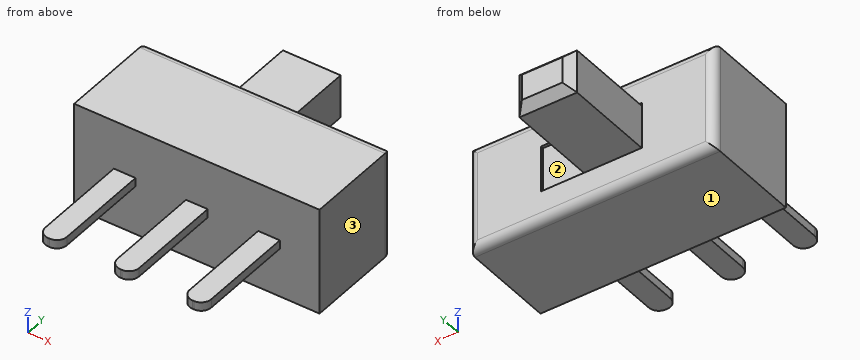
```python
from build123d import *

# Parameters (mm, degrees)
SKETCH1_W           = 8.5
SKETCH1_H           = 3.7
BOSS_EXTRUDE1_DEPTH = 1.75
SKETCH2_W           = 3.5
SKETCH2_H           = 1.6
CUT_EXTRUDE1_DEPTH  = 0.1
SKETCH3_W           = 2
SKETCH3_H           = 1.5
BOSS_EXTRUDE2_DEPTH = 3.5
SKETCH4_W           = 0.75
SKETCH4_H           = 0.3
BOSS_EXTRUDE3_DEPTH = 3.7
CHAMFER1_SIZE       = 0.3
FILLET1_R           = 0.3
FILLET2_R           = 0.35


with BuildPart() as part:
    # Sketch1 → Boss-Extrude1 (new, symmetric)
    with BuildSketch(Plane(origin=(0, 0, 0), x_dir=(1, 0, 0), z_dir=(0, 1, 0))):
        Rectangle(SKETCH1_W, SKETCH1_H)
    extrude(amount=BOSS_EXTRUDE1_DEPTH, both=True)

    # Sketch2 → Cut-Extrude1 (cut)
    with BuildSketch(Plane(origin=(0, 1.75, 0), x_dir=(1, 0, 0), z_dir=(0, 1, 0))):
        Rectangle(SKETCH2_W, SKETCH2_H)
    extrude(amount=-CUT_EXTRUDE1_DEPTH, mode=Mode.SUBTRACT)

    # Sketch3 → Boss-Extrude2 (add)
    with BuildSketch(Plane(origin=(0, 1.65, 0), x_dir=(1, 0, 0), z_dir=(0, 1, 0))):
        with Locations((-0.7, 0)):
            Rectangle(SKETCH3_W, SKETCH3_H)
    extrude(amount=BOSS_EXTRUDE2_DEPTH)

    # Sketch4 → Boss-Extrude3 (add)
    with BuildSketch(Plane.XZ.offset(1.75)):
        Rectangle(SKETCH4_W, SKETCH4_H)
        with Locations((-2.5, 0)):
            Rectangle(SKETCH4_W, SKETCH4_H)
        with Locations((2.5, 0)):
            Rectangle(SKETCH4_W, SKETCH4_H)
    extrude(amount=BOSS_EXTRUDE3_DEPTH)

    # Chamfer1
    chamfer1_edges = [part.edges().sort_by_distance(p)[0] for p in [
        (-1.7, 5.15, 0),
        (-0.7, 5.15, 0.75),
        (0.3, 5.15, 0),
        (-0.7, 5.15, -0.75),
    ]]
    chamfer(chamfer1_edges, length=CHAMFER1_SIZE)

    # Fillet1
    fillet1_edges = [part.edges().sort_by_distance(p)[0] for p in [
        (-4.25, 1.75, 0),
        (0, 1.75, 1.85),
        (4.25, 1.75, 0),
        (0, 1.75, -1.85),
    ]]
    fillet(fillet1_edges, radius=FILLET1_R)

    # Fillet2
    fillet2_edges = [part.edges().sort_by_distance(p)[0] for p in [
        (0.375, -5.45, 0),
        (-0.375, -5.45, 0),
        (-2.125, -5.45, 0),
        (-2.875, -5.45, 0),
        (2.125, -5.45, 0),
        (2.875, -5.45, 0),
    ]]
    fillet(fillet2_edges, radius=FILLET2_R)


solid = part.part
```
Design review of the part built by this model. Coordinates are the model's own, in mm. Face numbers are marked on the shaded views. Give positions to 0.01 mm unless a question says otherwise; leave off trailing zeros. Write each loop counter-clockwise with the first axis right and the second up, starting at its lowest first coordinate (ties: lowest second). Pieces come first, ordered by that corner, then holes. Notation, with made-up numbers: (74.5, 1) -> (94.5, 1) arc R22 ccw to (94.5, 35) -> close; hole circle Ø3 at (44, 44). An arc over 180 degrees is marked (long way). Answer in a Markdown table with one row per item.
(1) Consider section C-C (z = 0.6). State the section outline as (x, y) points.
Results:
| item | result |
|---|---|
| outline | (-4.25, -1.75) -> (4.25, -1.75) -> (4.25, 1.45) arc R0.3 ccw to (3.95, 1.75) -> (1.75, 1.75) -> (1.75, 1.65) -> (0.3, 1.65) -> (0.3, 4.85) -> (0.15, 5) -> (-1.55, 5) -> (-1.7, 4.85) -> (-1.7, 1.65) -> (-1.75, 1.65) -> (-1.75, 1.75) -> (-3.95, 1.75) arc R0.3 ccw to (-4.25, 1.45) -> close |
(2) Clearance check with flat-ended pins moving along their axes: pin 1 (0.6 mm diameter, centred on x = -1, y = 3, fed in from +Z); pin 2 (1.8 mm diameter, centred on x = -1, z = -0.5, fed in from -Y); pin 3 (0.6 mm diameter, centred on x = 2.5, y = -3, fed in from -Z). State where each tip first meets the part, or that it passes through.
Results:
| item | result |
|---|---|
| pin 1 | z = 0.75 |
| pin 2 | y = -5.42 |
| pin 3 | z = -0.15 |
(3) Consider section D-D (x = 0.75). State the section outline as (y, z) points.
Results:
| item | result |
|---|---|
| outline | (-1.75, -1.85) -> (1.45, -1.85) arc R0.3 ccw to (1.75, -1.55) -> (1.75, -0.8) -> (1.65, -0.8) -> (1.65, 0.8) -> (1.75, 0.8) -> (1.75, 1.55) arc R0.3 ccw to (1.45, 1.85) -> (-1.75, 1.85) -> close |
(4) Consider section B-B (x = -1.25). State the section outline as (y, z) points.
Results:
| item | result |
|---|---|
| outline | (-1.75, -1.85) -> (1.45, -1.85) arc R0.3 ccw to (1.75, -1.55) -> (1.75, -0.8) -> (1.65, -0.8) -> (1.65, -0.75) -> (4.85, -0.75) -> (5.15, -0.45) -> (5.15, 0.45) -> (4.85, 0.75) -> (1.65, 0.75) -> (1.65, 0.8) -> (1.75, 0.8) -> (1.75, 1.55) arc R0.3 ccw to (1.45, 1.85) -> (-1.75, 1.85) -> close |
(5) Consider section A-A (y = -2). State the section outline as (x, z) points (3 decimals).
Results:
| item | result |
|---|---|
| outline | (-2.875, -0.15) -> (-2.125, -0.15) -> (-2.125, 0.15) -> (-2.875, 0.15) -> close; (-0.375, -0.15) -> (0.375, -0.15) -> (0.375, 0.15) -> (-0.375, 0.15) -> close; (2.125, -0.15) -> (2.875, -0.15) -> (2.875, 0.15) -> (2.125, 0.15) -> close |
(6) Mouldability with a two-part tool opening along X and no side actions: class the marked faces 1, 2 and 3 as +X half, -X half, draft (parallel to the pull), parting line (faces both ways), or undercut.
Results:
| item | result |
|---|---|
| face 1 | draft |
| face 2 | undercut |
| face 3 | +X half |
(7) To check wall thickness, follow probe 1 along Y at (x, z) = (2, -1.45); probe 2 along Y at (x, z) = (-0.5, 0.4); probe 3 along X at (y, z) = (4.75, 0.45). State the ranges of each line that lie inside material, in increasing order.
Results:
| item | result |
|---|---|
| probe 1 | -1.75 to 1.75 |
| probe 2 | -1.75 to 5.15 |
| probe 3 | -1.7 to 0.3 |
